Source: CAD feature listing. Evaluate the final solid. Frame: model axes, mm. A direction names the side the tool comes from. Coordinates: 2 decimals unless noted, no trailing zeros. Write each loop counter-clockwise with the first axis right and the second up, starting at its lowest first coordinate (ties: lowest second). Pieces come first, ordered by that corner, then holes. Notation, with made-up numbers: (5, -21.75) -> (31, -21.75) arc R13 ccw to (31, -8.75) -> close; hole circle Ø8 at (86.5, 7). An arc over 180 degrees is marked (long way). One line per item, written item: value. Start each with the question number.
1. Section query B-B, the plane z = 41.5. Output: boundary loops of the cut face in (x, y).
2. Line query: line 1 (Y direction, x = 38.5, z = 12); line 2 (Z direction, x = 17, y = 2.5); line 3 (Z direction, x = -61, y = -6). Output: solid intervals per line, ascending.
3. Mould query, pull axis Z, two halves, no side actions, for faces 1 (the flat face through (-0.586, -36.175, 93.772)), 2 (the flat face through (19, -40.833, 4)). Classes: released by +Z, released by -Z, zero draft, split by the parting line, or undercut.
4. Access query for faces 3 (the flat face through (65.32, -38.42, 36.98)), 4 (the flat face through (-53.7, -22, 90.3)), 5 (the flat face through (0, -30.833, 4)). Directions: +Z, -Z, +X, -X, +Y, -Y. A direction counts if a zero-diameter tool reaches every point of the face in a straight line with its end or side. Return the directions, or none.
5. First-contact query: P1, Ø12, axis at x = -30.5, z = 46, coming from the +Y side; P2, Ø0.6, axis at x = -87.5, y = -0.5, coming from the -Z side; P3, Ø3, axis at x = -86, z = 44.5, coming from the +Y side; P4, Ø2.5, axis at y = -56, z = 4, coming from the -X side. Flat tips, straight axial feed; report the tip coordinate or a pass-through.
from build123d import *

# Parameters (mm, degrees)
F0_W      = 50
F0_H      = 12.5
F1_DEPTH  = 8
F2_DEPTH  = 75
F4_DEPTH  = 8
F7_DEPTH  = 3
F8_DEPTH  = 1
F11_DEPTH = 3
F14_DEPTH = 3
F15_DEPTH = 8
F16_DEPTH = 25


with BuildPart() as f1:
    # F0 (on Top) → F1 (new body)
    with BuildSketch(Plane.XY):
        Polygon((-42.017949, 72.777223), (-84.035898, 0), (-42.017949, -72.777223), (42.017949, -72.777223), (84.035898, 0), (42.017949, 72.777223), align=None)
        Polygon((25.132911, -40.832917), (25, -48.332917), (25, -60.832917), (-25, -60.832917), (-25, -48.332917), (-25, -40.832917), (-12.5, -40.832917), (-12.5, -30.832917), (12.566456, -30.832917), (12.566456, -40.832917), align=None, mode=Mode.SUBTRACT)
        with Locations((0, 54.582917)):
            Rectangle(F0_W, F0_H, mode=Mode.SUBTRACT)
    extrude(amount=F1_DEPTH)

    # F0 (on Top) → F2 (join)
    with BuildSketch(Plane.XY):
        Polygon((-84.035898, 0), (-87.5, 0), (-43.75, -75.777223), (43.75, -75.777223), (87.5, 0), (84.035898, 0), (42.017949, -72.777223), (-42.017949, -72.777223), align=None)
    extrude(amount=F2_DEPTH)

    # F0 (on Top) → F4 (join)
    with BuildSketch(Plane.XY):
        Polygon((43.75, 75.777223), (-43.75, 75.777223), (-87.5, 0), (-84.035898, 0), (-42.017949, 72.777223), (42.017949, 72.777223), (84.035898, 0), (87.5, 0), align=None)
    extrude(amount=F4_DEPTH)

    # F6 (on face) → F7 (join)
    with BuildSketch(Plane(origin=(0, -50.131237, 89.383668), x_dir=(1, 0, 0), z_dir=(0, 0.489171, -0.872188))):
        Polygon((43.75, 29.404192), (0, 29.404192), (-43.75, 29.404192), (-42.01795, -57.477552), (42.01795, -57.477552), align=None)
    extrude(amount=F7_DEPTH)

    # F3 (on Front) → F8 (join)
    with BuildSketch(Plane.XZ):
        Polygon((-42.01795, 114.5), (0, 114.5), (42.01795, 114.5), (84.0359, 75), (87.5, 75), (42.01795, 117.5), (0, 117.5), (-42.01795, 117.5), (-87.5, 75), (-84.0359, 75), align=None)
    extrude(amount=F8_DEPTH)

    # F10 (on face) → F11 (join)
    with BuildSketch(Plane(origin=(-67.684673, -39.077764, 72.433827), x_dir=(0.772363, -0.301588, 0.559017), z_dir=(-0.635181, -0.366722, 0.67975))):
        Polygon((33.231426, 55.789645), (-25.65546, 35.610412), (30.988892, -31.080422), align=None)
    extrude(amount=-F11_DEPTH)

    # F13 (on face) → F14 (join)
    with BuildSketch(Plane(origin=(67.675669, -39.595085, 72.424192), x_dir=(0.773305, 0.304147, -0.556322), z_dir=(-0.634035, 0.370955, -0.678522))):
        Polygon((-30.93951, 30.511739), (-32.875165, -56.364915), (25.940007, -35.977606), align=None)
    extrude(amount=F14_DEPTH)

    # F0 (on Top) → F15 (join)
    with BuildSketch(Plane.XY):
        with Locations((0, 54.582917)):
            Rectangle(F0_W, F0_H)
    extrude(amount=F15_DEPTH)

    # F0 (on Top) → F16 (cut)
    with BuildSketch(Plane.XY):
        Polygon((25, -60.832917), (25, -48.332917), (25.132911, -40.832917), (12.566456, -40.832917), (0, -40.832917), (-12.5, -40.832917), (-25, -40.832917), (-25, -48.332917), (-25, -60.832917), align=None)
    extrude(amount=-F16_DEPTH, mode=Mode.SUBTRACT)


solid = f1.part
Computed values:
1. outline: (-87.5, 0) -> (-43.75, -75.78) -> (43.75, -75.78) -> (87.5, 0) -> (84.04, 0) -> (42.02, -72.78) -> (-42.02, -72.78) -> (-84.04, 0) -> close
2. line 1: y = -75.78 to -72.78
2. line 2: z = 0 to 8
2. line 3: z = 0 to 8, 92.11 to 96.53
3. face 1: undercut
3. face 2: zero draft
4. face 3: -Z, +X, -Y
4. face 4: +Y
4. face 5: -Z
5. P1: stops at y = -72.78
5. P2: stops at z = 0
5. P3: stops at y = 0
5. P4: stops at x = -55.89
